```python
from build123d import *

# Parameters (mm, degrees)
ESQUISSE1_W             = 15
ESQUISSE1_H             = 15
BOSS_EXTRU_1_DEPTH      = 5
ESQUISSE2_R             = 1.5
ENL_V_MAT_EXTRU_1_DEPTH = 3
ESQUISSE3_W             = 13
ESQUISSE3_H             = 10.5
BOSS_EXTRU_2_DEPTH      = 2
ESQUISSE4_W             = 15
ESQUISSE4_H             = 12
BOSS_EXTRU_3_DEPTH      = 0.5
ESQUISSE5_R             = 3.05
ENL_V_MAT_EXTRU_2_DEPTH = 1
ESQUISSE5_3_R           = 3.05
ENL_V_MAT_EXTRU_3_DEPTH = 15


with BuildPart() as part:
    # Esquisse1 → Boss.-Extru.1 (new body)
    with BuildSketch(Plane.XY):
        Rectangle(ESQUISSE1_W, ESQUISSE1_H)
    extrude(amount=BOSS_EXTRU_1_DEPTH)

    # Esquisse2 → Enl_v. mat.-Extru.1 (cut)
    with BuildSketch(Plane(origin=(0, 7.5, 0), x_dir=(1, 0, 0), z_dir=(0, 1, 0))):
        with Locations(Location((0, -2.5, 0), (0, 0, 270))):
            Circle(ESQUISSE2_R)
    extrude(amount=-ENL_V_MAT_EXTRU_1_DEPTH, mode=Mode.SUBTRACT)

    # Esquisse3 → Boss.-Extru.2 (add)
    with BuildSketch(Plane(origin=(0, 0, 0), x_dir=(-1, 0, 0), z_dir=(0, 0, -1))):
        with Locations((0, -2.25)):
            Rectangle(ESQUISSE3_W, ESQUISSE3_H)
    extrude(amount=BOSS_EXTRU_2_DEPTH)

    # Esquisse4 → Boss.-Extru.3 (add)
    with BuildSketch(Plane(origin=(0, 0, -2), x_dir=(-1, 0, 0), z_dir=(0, 0, -1))):
        with Locations((0, -1.5)):
            Rectangle(ESQUISSE4_W, ESQUISSE4_H)
    extrude(amount=BOSS_EXTRU_3_DEPTH)

    # Esquisse5 → Enl_v. mat.-Extru.2 (cut)
    with BuildSketch(Plane(origin=(0, 0, -2.5), x_dir=(-1, 0, 0), z_dir=(0, 0, -1))):
        with Locations((0, -1)):
            Circle(ESQUISSE5_R)
    extrude(amount=-ENL_V_MAT_EXTRU_2_DEPTH, mode=Mode.SUBTRACT)

    # Esquisse5_3 → Enl_v. mat.-Extru.3 (cut)
    with BuildSketch(Plane(origin=(0, 0, -2.5), x_dir=(-1, 0, 0), z_dir=(0, 0, -1))):
        with Locations((0, -1)):
            Circle(ESQUISSE5_3_R)
    extrude(amount=-ENL_V_MAT_EXTRU_3_DEPTH, mode=Mode.SUBTRACT)


solid = part.part
```
Could you check a few things on this model? Use its own coordinates, in mm. A direction names the side the tool comes from. Round coordinates to 2 decimals unless told otherwise and drop trailing zeros. Write each loop counter-clockwise with the first axis right and the second up, starting at its lowest first coordinate (ties: lowest second). Pieces come first, ordered by that corner, then holes.
(1) If I drill on probe 1 along X at (y, z) = (5.55, 2.5); probe 2 along Z at (x, y) = (1, 3.5); probe 3 along X at (y, z) = (-0.25, 4), over which ranges is the centre line in solid material (lowest first)?
Findings below:
probe 1: x = -7.5 to -1.5, 1.5 to 7.5
probe 2: z = -2.5 to -2, 0 to 5
probe 3: x = -7.5 to -2.96, 2.96 to 7.5
(2) Suppose I cut it at D-D on x = 6. Write out the boundary of the cut face in (y, z).
Findings below:
outline: (-7.5, -2.5) - (4.5, -2.5) - (4.5, -2) - (3, -2) - (3, 0) - (7.5, 0) - (7.5, 5) - (-7.5, 5) - close
(3) Thinking about a two-plate mould opening in X: for faces 5 (the face through (-6.5, -2, -1)), 6 (the face through (0.397, 2.024, 1.197)), 7 (the face through (2, -4, -2.5)), which applies, +X half, -X half, draft (parallel to the pull), parting line (faces both ways), or undercut?
Findings below:
face 5: -X half
face 6: undercut
face 7: draft
(4) Suppose I cut it at B-B on y = -1. Write out the boundary of the cut face in (x, z), and give its area (4 significant figures).
Findings below:
outline: (-7.5, -2.5) - (-3.05, -2.5) - (-3.05, 5) - (-7.5, 5) - (-7.5, 0) - (-6.5, 0) - (-6.5, -2) - (-7.5, -2) - close; (3.05, -2.5) - (7.5, -2.5) - (7.5, -2) - (6.5, -2) - (6.5, 0) - (7.5, 0) - (7.5, 5) - (3.05, 5) - close
area: 62.75 mm2
(5) For pin 1 (5 mm diameter, centred on x = 0, y = -1, fed in from +Z); pin 2 (1.6 mm diameter, centred on y = -3.5, z = -1, fed in from +X); pin 3 (2 mm diameter, centred on x = -2, z = -1.5, fed in from +Y), each with a flat end and sliding along its axis, tell me the tip position at first contact or that it passes through.
Findings below:
pin 1: passes through
pin 2: stops at x = 6.5
pin 3: stops at y = 4.5
(6) Suppose I cut it at C-C on z = 2.5. Write out the boundary of the cut face in (x, y).
Findings below:
outline: (-7.5, -7.5) - (7.5, -7.5) - (7.5, 7.5) - (1.5, 7.5) - (1.5, 4.5) - (-1.5, 4.5) - (-1.5, 7.5) - (-7.5, 7.5) - close; hole circle Ø6.1 at (0, -1)
(7) Which directions (+Z, -Z, +X, -X, +Y, -Y) give clear straight access to the entire face, cutting with the end or side of a thin tool? Please do faces 1 (the face through (-0.1, 3.4, 0)), 2 (the face through (0, 3, -1)), 3 (the face through (-2, 2, 5)), 4 (the face through (6.5, -2, -1)).
Findings below:
face 1: +Y
face 2: +X, -X, +Y
face 3: +Z, +X, -X, +Y, -Y
face 4: +X, +Y, -Y
(8) Suppose I cut it at A-A on x = 0. Write out the boundary of the cut face in (y, z), and give its area (4 significant figures).
Findings below:
outline: (-7.5, -2.5) - (-4.05, -2.5) - (-4.05, 5) - (-7.5, 5) - close; (2.05, -2.5) - (4.5, -2.5) - (4.5, -2) - (3, -2) - (3, 0) - (7.5, 0) - (7.5, 1) - (4.5, 1) - (4.5, 4) - (7.5, 4) - (7.5, 5) - (2.05, 5) - close
area: 47.25 mm2
